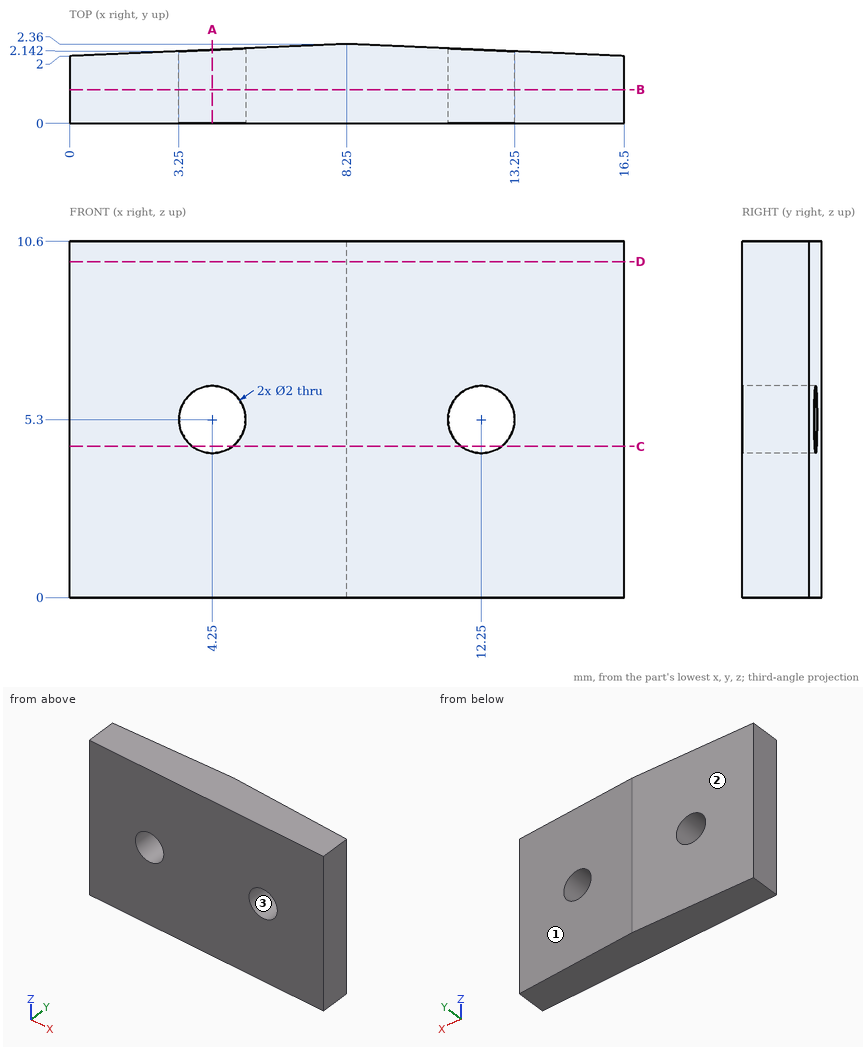
Geometry: see drawing. Coordinates: mm, zero at the bounding-box minimum. Coordinates: 2 decimals unless noted, no trailing zeros. Loops run counter-clockwise (first coordinate to the right, second up) from the corner with the lowest first, then second, coordinate; pieces in that order, holes last. Notation, with made-up numbers: (15.5, 0) - (63.5, 0) arc R12 ccw to (63.5, 19) - close; hole circle Ø6 at (79.25, -2.75). An arc over 180 degrees is marked (long way). Put each result on its own line as item: value. Start each with the question number.
Q1. Cut plane C-C, the plane z = 4.5. Return loops of the section in (x, y), and give its area (3 significant figures).
Q2. Cut plane D-D, the plane z = 10. Return loops of the section in (x, y), and give its area (3 significant figures).
Q3. Cut plane B-B, the plane y = 1. Return loops of the section in (x, z), and give its area (3 significant figures).
Q4. Pin query (flat end, axial travel): pin 1 Ø1.8 at (x, z) = (12.25, 5.3) entering from +Y; pin 2 Ø2.5 at (x, z) = (4.25, 5.3) entering from +Y. Return the tip coordinate at first contact, or that it passes through.
Q5. Cut plane A-A, the plane x = 4.25. Return loops of the section in (y, z), and give its area (3 significant figures).
Q6. Line query: line 1 (Z direction, x = 12.25, y = 1.7); line 2 (X direction, y = 1, z = 5.3); line 3 (Y direction, x = 11.25, z = 1.25). Output: solid intervals per line, ascending.
Q7. Pull-direction query (X, two-part tool) for the marked faces 1, 2 and 3; classes: released by +X, released by -X, zero draft, split by the parting line, or undercut.
Filled sheet:
1. outline: (0, 0) - (3.65, 0) - (3.65, 2.16) - (0, 2) - close; (4.85, 0) - (11.65, 0) - (11.65, 2.21) - (8.25, 2.36) - (4.85, 2.21) - close; (12.85, 0) - (16.5, 0) - (16.5, 2) - (12.85, 2.16) - close
1. area: 30.7 mm²
2. outline: (0, 0) - (16.5, 0) - (16.5, 2) - (8.25, 2.36) - (0, 2) - close
2. area: 36.0 mm²
3. outline: (0, 0) - (16.5, 0) - (16.5, 10.6) - (0, 10.6) - close; hole circle Ø2 at (4.25, 5.3); hole circle Ø2 at (12.25, 5.3)
3. area: 169 mm²
4. pin 1: through
4. pin 2: y = 2.24
5. outline: (0, 0) - (2.19, 0) - (2.19, 4.3) - (0, 4.3) - close; (0, 6.3) - (2.19, 6.3) - (2.19, 10.6) - (0, 10.6) - close
5. area: 18.8 mm²
6. line 1: 0 to 4.3, 6.3 to 10.6
6. line 2: 0 to 3.25, 5.25 to 11.25, 13.25 to 16.5
6. line 3: 0 to 2.23
7. face 1: released by +X
7. face 2: released by -X
7. face 3: undercut
